Check sheet for the drawn part. Datum: minimum x, y, z corner. Units: mm. A direction names the side the tool comes from. Round coordinates to 2 decimals unless told otherwise and drop trailing zeros. Write each loop counter-clockwise with the first axis right and the second up, starting at its lowest first coordinate (ties: lowest second). Pieces come first, ordered by that corner, then holes. Notation, with made-up numbers: (54.5, 72) - (101.5, 72) arc R15 ccw to (101.5, 83) - close; hole circle Ø4 at (-29, -38.75). An arc over 180 degrees is marked (long way). Answer as a JSON object with one key per item and string values.
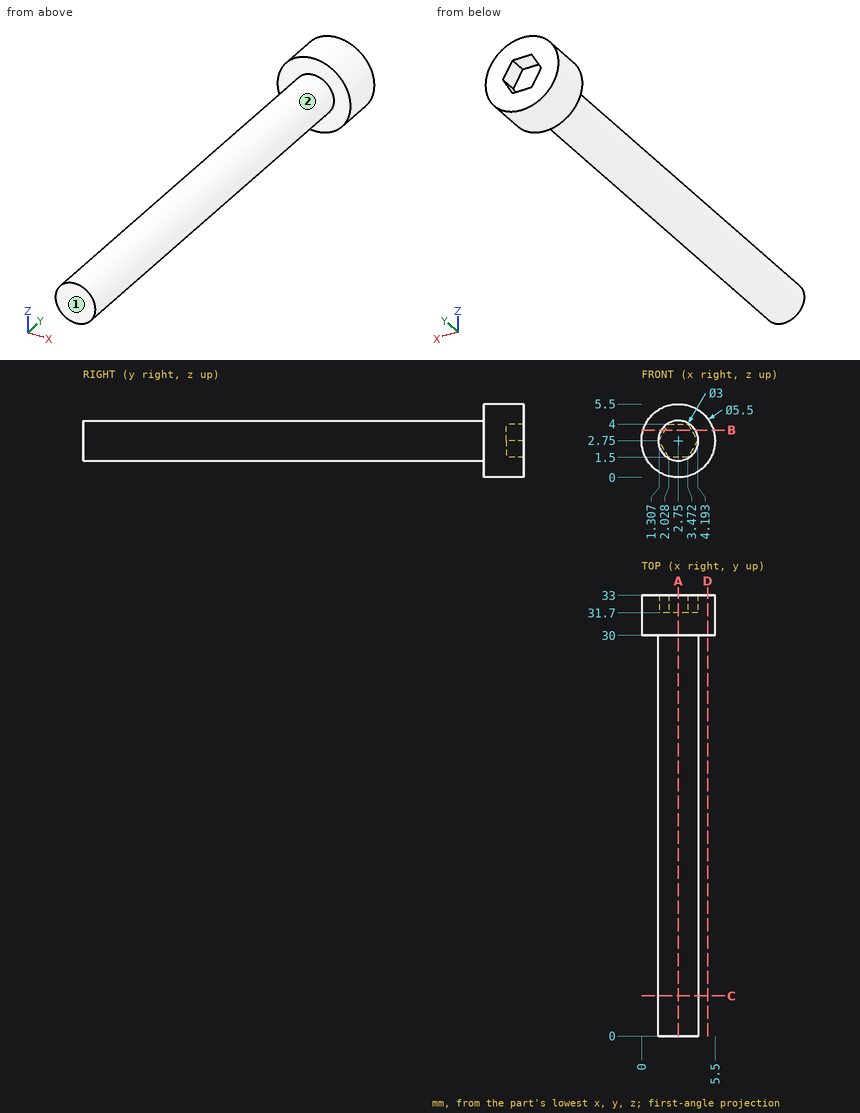
Q1. Section check B-B, the plane z = 3.55. Record the cut outline in (x, y).
Geometry check:
{"outline": "(0.12, 30) - (1.48, 30) - (1.48, 0) - (4.02, 0) - (4.02, 30) - (5.38, 30) - (5.38, 33) - (3.73, 33) - (3.73, 31.7) - (1.77, 31.7) - (1.77, 33) - (0.12, 33) - close"}
Q2. Section check D-D, the plane x = 4.95. Record the cut outline in (y, z).
Geometry check:
{"outline": "(30, 1.1) - (33, 1.1) - (33, 4.4) - (30, 4.4) - close"}
Q3. Section check C-C, the plane y = 3. Record the cut outline in (x, z).
Geometry check:
{"outline": "circle Ø3 at (2.75, 2.75)"}
Q4. Material ranges on line 1 along Y through (x, z) = (4, 1.4); line 2 along X through (y, z) = (25, 2.35) (1 decimal); line 3 along Y through (x, z) = (3.05, 2.6), recorded low to high. Write a range as [from, to].
Geometry check:
{"line 1": "y = [30, 33]", "line 2": "x = [1.3, 4.2]", "line 3": "y = [0, 31.7]"}
Q5. Set-up check for the marked faces 1 and 2: record each of +Z, -Z, +X, -X, +Y, -Y from which the full face is reachable in a straight line by a thin tool's end or side.
Geometry check:
{"face 1": "+Z, -Z, +X, -X, -Y", "face 2": "-Y"}
Q6. Section check A-A, the plane x = 2.75. Record the cut outline in (y, z).
Geometry check:
{"outline": "(0, 1.25) - (30, 1.25) - (30, 0) - (33, 0) - (33, 1.5) - (31.7, 1.5) - (31.7, 4) - (33, 4) - (33, 5.5) - (30, 5.5) - (30, 4.25) - (0, 4.25) - close"}
Q7. Gauge pin test, flat ends, axial feed: P1, Ø1.5, axis at x = 1, z = 1, coming from the -Y side; P2, Ø1, axis at y = 21.5, z = 3.5, coming from the +X side; P3, Ø2, axis at y = 20, z = 1, coming from the -X side. Record the tip position at first contact, or that the pin passes through.
Geometry check:
{"P1": "stops at y = 30", "P2": "stops at x = 4.23", "P3": "stops at x = 1.45"}
